```python
from build123d import *

# Parameters (mm, degrees)
BOSS_EXTRUDE1_DEPTH = 23.3
SKETCH2_W           = 20
SKETCH2_H           = 10
SKETCH2_R           = 2
BOSS_EXTRUDE2_DEPTH = 5
FILLET1_START       = -1
FILLET1_DEPTH       = 6
FILLET1_2_DEPTH     = 5
SKETCH3_R           = 2.25
CUT_EXTRUDE1_DEPTH  = 124


with BuildPart() as part:
    # Sketch1 → Boss-Extrude1 (new body)
    with BuildSketch(Plane.XY):
        Polygon((-39.4, -14), (-39.4, 0), (39.4, 0), (39.4, -14), (34.4, -14), (34.4, -5), (-34.4, -5), (-34.4, -14), align=None)
    extrude(amount=BOSS_EXTRUDE1_DEPTH)

    # Sketch2 → Boss-Extrude2 (add)
    with BuildSketch(Plane(origin=(0, 0, 0), x_dir=(-1, 0, 0), z_dir=(0, 0, -1))):
        with Locations((0, 5)):
            Rectangle(SKETCH2_W, SKETCH2_H)
        with Locations((5, 5)):
            Circle(SKETCH2_R, mode=Mode.SUBTRACT)
        with Locations(Location((-5, 5, 0), (0, 0, 180))):
            Circle(SKETCH2_R, mode=Mode.SUBTRACT)
    extrude(amount=-BOSS_EXTRUDE2_DEPTH)

    # Fillet1: read off the stored shape, not the designer's step
    # Fillet1 outline → Fillet1 (cut)
    with BuildSketch(Plane.XY.offset(FILLET1_START)):
        with BuildLine():
            Line((-10, 10), (-10, 5))
            ThreePointArc((-10, 5), (-8.535533906, 8.535533906), (-5, 10))
            Line((-5, 10), (-10, 10))
        make_face()
        with BuildLine():
            Line((10, 10), (5, 10))
            ThreePointArc((5, 10), (8.535533906, 8.535533906), (10, 5))
            Line((10, 5), (10, 10))
        make_face()
    extrude(amount=FILLET1_DEPTH, mode=Mode.SUBTRACT)

    # Fillet1 2 outline → Fillet1 2 (add)
    with BuildSketch(Plane.XY):
        with BuildLine():
            Line((-10, 0), (-10, 5))
            ThreePointArc((-10, 5), (-11.464466094, 1.464466094), (-15, 0))
            Line((-15, 0), (-10, 0))
        make_face()
        with BuildLine():
            Line((10, 5), (10, 0))
            Line((10, 0), (15, 0))
            ThreePointArc((15, 0), (11.464466094, 1.464466094), (10, 5))
        make_face()
    extrude(amount=FILLET1_2_DEPTH)

    # Sketch3 → Cut-Extrude1 (cut)
    with BuildSketch(Plane(origin=(39.4, 0, 0), x_dir=(0, 0, -1), z_dir=(1, 0, 0))):
        with Locations((-4.55, -10)):
            Circle(SKETCH3_R)
        with Locations((-14.55, -10)):
            Circle(SKETCH3_R)
    extrude(amount=-CUT_EXTRUDE1_DEPTH, mode=Mode.SUBTRACT)


solid = part.part
```
Geometry check sheet. Reference: the model listing, model coordinates, mm. A direction names the side the tool comes from. Coordinates: 2 decimals unless noted, no trailing zeros. Loops run counter-clockwise (first coordinate to the right, second up) from the corner with the lowest first, then second, coordinate; pieces in that order, holes last. Notation, with made-up numbers: (-21.75, -23.75) - (-5.75, -23.75) arc R22 ccw to (-5.75, 4.25) - close; hole circle Ø2 at (82, -8.5). An arc over 180 degrees is marked (long way). One line per item, written item: value. Start each with the question number.
(1) Material ranges on line 1 (Y direction, x = 5, z = 2.2); line 2 (X direction, y = -6.5, z = 13.5); line 3 (Y direction, x = 38.15, z = 4.55), recorded low to high. Write a range as [from, to].
(2) Tool access check on faces 1 (the flat face through (39.4, -7, 11)), 2 (the flat face through (34.4, -10, 11)), 3 (the flat face through (0, 5, 5)). Record the directions out of +Z, -Z, +X, -X, +Y, -Y that give a thin tool (end or side, any length) a straight path to the whole face; none if there is none.
(3) Cross-section at A-A on y = -10. Enter the section's corners in (x, z), plus the area to 3 significant figures.
(4) Cross-section at B-B on z = 13.5. Enter the section's corners in (x, y).
(5) Depth check by flat-ended pin: P1, Ø11.5, axis at x = 17, z = 13.5, coming from the -Y side; P2, Ø4, axis at y = -10, z = 14.55, coming from the +X side; P3, Ø10, axis at x = -1, z = 16, coming from the +Y side; P4, Ø2, axis at x = 7.5, z = 3, coming from the +Y side. Enter the tip coordinate at first touch or a pass-through.
(6) Cross-section at D-D on x = -13.5. Enter the section's corners in (y, z), plus the area to 3 significant figures.
(7) Mould release check, pull along Y, two halves, no side actions. Record for faces 4 (the cylindrical face through (36.94, -8.48, 16.21)), 5 (the flat face through (0, -5, 11)), 6 (the flat face through (0, 10, 2)), 7 (the flat face through (-39.4, -7, 11)): released by +Y, released by -Y, zero draft, split by the parting line, or undercut.
(8) Cross-section at C-C on z = 20. Enter the section's corners in (x, y).
Results below:
1. line 1: y = [-5, 3], [7, 10]
1. line 2: x = [-39.4, -34.4], [34.4, 39.4]
1. line 3: y = [-14, -12.25], [-7.75, 0]
2. face 1: +Z, -Z, +X, +Y, -Y
2. face 2: +Z, -Z, -Y
2. face 3: +Z, +X, -X, +Y
3. outline: (-39.4, 0) - (-34.4, 0) - (-34.4, 2.3) - (-39.4, 2.3) - close; (-39.4, 6.8) - (-34.4, 6.8) - (-34.4, 12.3) - (-39.4, 12.3) - close; (-39.4, 16.8) - (-34.4, 16.8) - (-34.4, 23.3) - (-39.4, 23.3) - close; (34.4, 0) - (39.4, 0) - (39.4, 2.3) - (34.4, 2.3) - close; (34.4, 6.8) - (39.4, 6.8) - (39.4, 12.3) - (34.4, 12.3) - close; (34.4, 16.8) - (39.4, 16.8) - (39.4, 23.3) - (34.4, 23.3) - close
3. area: 143 mm2
4. outline: (-39.4, -14) - (-34.4, -14) - (-34.4, -11.99) - (-39.4, -11.99) - close; (-39.4, -8.01) - (-34.4, -8.01) - (-34.4, -5) - (34.4, -5) - (34.4, -8.01) - (39.4, -8.01) - (39.4, 0) - (-39.4, 0) - close; (34.4, -14) - (39.4, -14) - (39.4, -11.99) - (34.4, -11.99) - close
5. P1: stops at y = -5
5. P2: passes through
5. P3: stops at y = 0
5. P4: stops at y = 9.77
6. outline: (-5, 0) - (0.23, 0) - (0.23, 5) - (0, 5) - (0, 23.3) - (-5, 23.3) - close
6. area: 118 mm2
7. face 4: undercut
7. face 5: released by -Y
7. face 6: released by +Y
7. face 7: zero draft
8. outline: (-39.4, -14) - (-34.4, -14) - (-34.4, -5) - (34.4, -5) - (34.4, -14) - (39.4, -14) - (39.4, 0) - (-39.4, 0) - close
